Verification items for the finished model (mm, model axes). Face numbers are marked on the shaded views. Round coordinates to 2 decimals unless told otherwise and drop trailing zeros. Write each loop counter-clockwise with the first axis right and the second up, starting at its lowest first coordinate (ties: lowest second). Pieces come first, ordered by that corner, then holes. Notation, with made-up numbers: (-14, 49) -> (23, 49) arc R30 ccw to (23, 81) -> close; hole circle Ø5 at (89.25, 26.5). An arc over 180 degrees is marked (long way). Use CSV: the item, a comma, the result in double quotes.
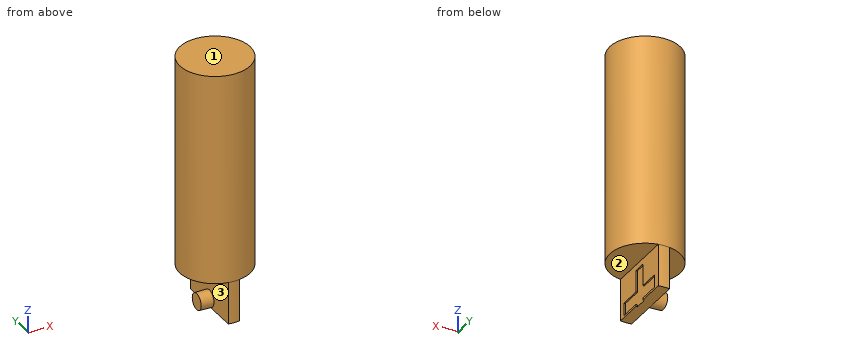
```python
from build123d import *

# Parameters (mm, degrees)
ESQUISSE1_R             = 25
BOSS_EXTRU_1_DEPTH      = 150
BOSS_EXTRU_2_START      = 30
BOSS_EXTRU_2_DEPTH      = 30
ESQUISSE3_R             = 6
BOSS_EXTRU_3_DEPTH      = 9
BOSS_EXTRU_3_TAPER      = 1
ENL_V_MAT_EXTRU_1_DEPTH = 1


with BuildPart() as part:
    # Esquisse1 → Boss.-Extru.1 (new body)
    with BuildSketch(Plane.XY):
        Circle(ESQUISSE1_R)
    extrude(amount=BOSS_EXTRU_1_DEPTH)

    # Esquisse2 → Boss.-Extru.2 (add)
    with BuildSketch(Plane(origin=(0, 0, 0), x_dir=(-1, 0, 0), z_dir=(0, 0, -1)).offset(BOSS_EXTRU_2_START)):
        with BuildLine():
            Line((-4, -24.677925359), (-4, 24.677925359))
            ThreePointArc((-4, 24.677925359), (0, 25), (4, 24.677925359))
            Line((4, 24.677925359), (4, -24.677925359))
            ThreePointArc((4, -24.677925359), (0, -25), (-4, -24.677925359))
        make_face()
    extrude(amount=-BOSS_EXTRU_2_DEPTH)

    # Esquisse3 → Boss.-Extru.3 (add)
    with BuildSketch(Plane.ZY.offset(4)):
        with Locations((-24, 0)):
            Circle(ESQUISSE3_R)
    extrude(amount=BOSS_EXTRU_3_DEPTH, taper=BOSS_EXTRU_3_TAPER)

    # Esquisse4 → Enlèv. mat.-Extru.1 (cut)
    with BuildSketch(Plane(origin=(4, 0, 0), x_dir=(0, 0, -1), z_dir=(1, 0, 0))):
        Polygon((19.5, 4.5), (19.5, 20), (28.5, 20), (28.5, 4.5), (30, 4.5), (30, -4.5), (28.5, -4.5), (28.5, -20), (19.5, -20), (19.5, -4.5), (4, -4.5), (4, 4.5), align=None)
    extrude(amount=-ENL_V_MAT_EXTRU_1_DEPTH, mode=Mode.SUBTRACT)


solid = part.part
```
Q1. Mould release check, pull along Z, two halves, no side actions. Record for the marked faces 1, 2 and 3: released by +Z, released by -Z, zero draft, split by the parting line, or undercut.
Filled in:
face 1,"released by +Z"
face 2,"released by -Z"
face 3,"undercut"
Q2. Section check B-B (y = -17.5). Record the cut outline in (x, z), plus the area to 3 significant figures.
Filled in:
outline,"(-17.85, 0) -> (-4, 0) -> (-4, -30) -> (4, -30) -> (4, -28.5) -> (3, -28.5) -> (3, -19.5) -> (4, -19.5) -> (4, 0) -> (17.85, 0) -> (17.85, 150) -> (-17.85, 150) -> close"
area,"5,590 mm²"
Q3. Section check C-C (z = 121). Record the cut outline in (x, y), plus the area to 3 significant figures.
Filled in:
outline,"circle Ø50 at (0, 0)"
area,"1,960 mm²"
Q4. Section check A-A (x = -10). Record the cut outline in (y, z), plus the area to 3 significant figures.
Filled in:
outline,"(-22.91, 0) -> (22.91, 0) -> (22.91, 150) -> (-22.91, 150) -> close; circle Ø11.79 at (0, -24)"
area,"6,980 mm²"
Q5. Section check D-D (y = -10). Record the cut outline in (x, z).
Filled in:
outline,"(-22.91, 0) -> (-4, 0) -> (-4, -30) -> (4, -30) -> (4, -28.5) -> (3, -28.5) -> (3, -19.5) -> (4, -19.5) -> (4, 0) -> (22.91, 0) -> (22.91, 150) -> (-22.91, 150) -> close"
Q6. Go/stop test with flat-tipped pins: P1, Ø0.8, axis at x = 3.5, y = 0.5, coming from the -Z side; P2, Ø17, axis at x = 15.5, y = 11, coming from the -Z side; P3, Ø4, axis at x = -8, y = -2, coming from the -Z side. Record where each tip stops, or that it passes through.
Filled in:
P1,"z = -4"
P2,"z = 0"
P3,"z = -29.94"
Q7. Material ranges on L1, parallel to Z at x = -10.5, y = 0.5; L2, parallel to X at y = 4, z = 61; L3, parallel to Z at x = -8, y = 17.5, recorded low to high.
Filled in:
L1,"-29.87 to -18.13, 0 to 150"
L2,"-24.68 to 24.68"
L3,"0 to 150"
